CAD build for the part. Positions are in the model's coordinates, mm. Give positions to 0.01 mm unless a question says otherwise; leave off trailing zeros. Order: outer loops, then holes, each group sorted by start corner. A loop starts at its lowest first (then second) coordinate and runs counter-clockwise, first axis right, second up.
Item 1: Band-saw the part on D-D on y = -17. Give the cut face in (x, z).
Item 2: Band-saw the part on B-B on z = 0. Give the cut face in (x, y) (1 decimal), plus the area to 3 significant figures.
Item 3: Two-plate mould, pull along Y, no slides. Class faces 1 (the cylindrical face through (1.97, -13.43, 11.45)), 2 (the flat face through (4, 0, -5)), 3 (the cylindrical face through (1.972, 22.804, 2.994)): released by +Y, released by -Y, zero draft, split by the parting line, or undercut.
Item 4: Band-saw the part on C-C on y = 14. Give the cut face in (x, z).
Item 5: Flat gauge pins, fed straight in: P1, Ø2, axis at x = 1, y = 9, coming from the +Z side; P2, Ø2, axis at x = 3.5, z = 9, coming from the +Y side; P3, Ø1.2, axis at x = 1, y = 10.5, coming from the -Z side. Where does each tip first touch, or does it go through?
Item 6: Wall check: L1, parallel to Y at x = 2.6, z = 0 (1 decimal); L2, parallel to Y at x = 2.75, z = -9; L3, parallel to Y at x = 1.55, z = 16. Give the ranges that are in metal, low to high.
Item 7: Band-saw the part on A-A on y = 0. Give the cut face in (x, z) (1 decimal), plus the area to 3 significant figures.
```python
from build123d import *

# Parameters (mm, degrees)
SKETCH1_R           = 23
SKETCH1_R_2         = 3.175
BOSS_EXTRUDE1_DEPTH = 4


with BuildPart() as part:
    # Sketch1 → Boss-Extrude1 (new body)
    with BuildSketch(Plane(origin=(0, 0, 0), x_dir=(0, 0, -1), z_dir=(1, 0, 0))):
        Circle(SKETCH1_R)
        Circle(SKETCH1_R_2, mode=Mode.SUBTRACT)
        with Locations((0, 18.5125)):
            Circle(SKETCH1_R_2, mode=Mode.SUBTRACT)
        with Locations((16.032295288, -9.25625)):
            Circle(SKETCH1_R_2, mode=Mode.SUBTRACT)
        with Locations((-16.032295288, -9.25625)):
            Circle(SKETCH1_R_2, mode=Mode.SUBTRACT)
        with BuildLine():
            Line((6, 2.309401077), (15.451717731, -3.1475507))
            ThreePointArc((15.451717731, -3.1475507), (17.376490414, -3.188857015), (18.444355761, -1.586945753))
            ThreePointArc((18.444355761, -1.586945753), (16.032295288, 9.25625), (7.847842544, 16.766753522))
            ThreePointArc((7.847842544, 16.766753522), (5.926614023, 16.642910634), (5, 14.955355437))
            Line((5, 14.955355437), (5, 4.041451884))
            ThreePointArc((5, 4.041451884), (5.267949192, 3.041451884), (6, 2.309401077))
        make_face(mode=Mode.SUBTRACT)
        with BuildLine():
            Line((-5, 4.041451884), (-5, 14.955355437))
            ThreePointArc((-5, 14.955355437), (-5.926614023, 16.642910634), (-7.847842544, 16.766753522))
            ThreePointArc((-7.847842544, 16.766753522), (-16.032295288, 9.25625), (-18.444355761, -1.586945753))
            ThreePointArc((-18.444355761, -1.586945753), (-17.376490414, -3.188857015), (-15.451717731, -3.1475507))
            Line((-15.451717731, -3.1475507), (-6, 2.309401077))
            ThreePointArc((-6, 2.309401077), (-5.267949192, 3.041451884), (-5, 4.041451884))
        make_face(mode=Mode.SUBTRACT)
        with BuildLine():
            Line((-1, -6.350852961), (-10.451717731, -11.807804737))
            ThreePointArc((-10.451717731, -11.807804737), (-11.449876391, -13.454053619), (-10.596513217, -15.179807769))
            ThreePointArc((-10.596513217, -15.179807769), (0, -18.5125), (10.596513217, -15.179807769))
            ThreePointArc((10.596513217, -15.179807769), (11.449876391, -13.454053619), (10.451717731, -11.807804737))
            Line((10.451717731, -11.807804737), (1, -6.350852961))
            ThreePointArc((1, -6.350852961), (0, -6.082903769), (-1, -6.350852961))
        make_face(mode=Mode.SUBTRACT)
    extrude(amount=BOSS_EXTRUDE1_DEPTH)


solid = part.part
```
The answers:
1. outline: (0, -15.49) - (4, -15.49) - (4, -7.33) - (0, -7.33) - close; (0, 7.33) - (4, 7.33) - (4, 15.49) - (0, 15.49) - close
2. outline: (0, -23) - (4, -23) - (4, -18.5) - (0, -18.5) - close; (0, -6.1) - (4, -6.1) - (4, -3.2) - (0, -3.2) - close; (0, 3.2) - (4, 3.2) - (4, 15.3) - (0, 15.3) - close; (0, 21.7) - (4, 21.7) - (4, 23) - (0, 23) - close
2. area: 83.5 mm2
3. face 1: undercut
3. face 2: zero draft
3. face 3: split by the parting line
4. outline: (0, -18.25) - (4, -18.25) - (4, -12.11) - (0, -12.11) - close; (0, -5) - (4, -5) - (4, 5) - (0, 5) - close; (0, 12.11) - (4, 12.11) - (4, 18.25) - (0, 18.25) - close
5. P1: stops at z = 21.56
5. P2: stops at y = 21.56
5. P3: stops at z = -20.76
6. L1: y = -23 to -18.5, -6.1 to -3.2, 3.2 to 15.3, 21.7 to 23
6. L2: y = -21.17 to -16.18, -10.97 to 0.58, 16.18 to 21.17
6. L3: y = -16.52 to -12.43, -6.08 to -3.36, 9.31 to 16.52
7. outline: (0, -23) - (4, -23) - (4, -18.5) - (0, -18.5) - close; (0, -10) - (4, -10) - (4, -3.2) - (0, -3.2) - close; (0, 3.2) - (4, 3.2) - (4, 10) - (0, 10) - close; (0, 18.5) - (4, 18.5) - (4, 23) - (0, 23) - close
7. area: 90.5 mm2
